```python
from build123d import *

# Parameters (mm, degrees)
EXTRUDE_1_DEPTH     = 8
SKETCH_2_R          = 1.5
CUT_EXTRUDE_1_DEPTH = 13.074353161
CHAMFER_1_SIZE      = 2


with BuildPart() as part:
    # ｽｹｯﾁ1 → ﾎﾞｽ - 押し出し1 (new body)
    with BuildSketch(Plane.XY):
        Polygon((-6.990630221, 0), (-3.009369779, 0), (-1.990630221, -2.4), (1.990630221, -2.4), (3.009369779, 0), (6.990630221, 0), (8.009369779, -2.4), (8.009369779, -4.2), (-8.009369779, -4.2), (-8.009369779, -2.4), align=None)
    extrude(amount=EXTRUDE_1_DEPTH)

    # ｽｹｯﾁ2 → ｶｯﾄ - 押し出し1 (cut, through all)
    with BuildSketch(Plane(origin=(0, 0, 0), x_dir=(1, 0, 0), z_dir=(0, 1, 0))):
        with Locations(Location((-5, -4, 0), (0, 0, 180))):
            Circle(SKETCH_2_R)
        with Locations(Location((5, -4, 0), (0, 0, 180))):
            Circle(SKETCH_2_R)
    extrude(amount=-CUT_EXTRUDE_1_DEPTH, mode=Mode.SUBTRACT)

    # 面取り1
    # the kernel refuses this chamfer: 2 mm, written as the material it takes off along each edge
    with BuildSketch(Plane(origin=(-5, -4.2, 4), x_dir=(-1, 0, 0), z_dir=(0, 0, -1))) as chamfer_1_piece_1:
        Polygon((1.5, CHAMFER_1_SIZE), (1.5 + CHAMFER_1_SIZE, 0), (1.5, 0), align=None)
    revolve(axis=Axis((-5, -4.2, 4), (0, 1, 0)), mode=Mode.SUBTRACT)
    with BuildSketch(Plane(origin=(5, -4.2, 4), x_dir=(-1, 0, 0), z_dir=(0, 0, -1))) as chamfer_1_piece_2:
        Polygon((1.5 + CHAMFER_1_SIZE, 0), (1.5, CHAMFER_1_SIZE), (1.5, 0), align=None)
    revolve(axis=Axis((5, -4.2, 4), (0, 1, 0)), mode=Mode.SUBTRACT)


solid = part.part
```
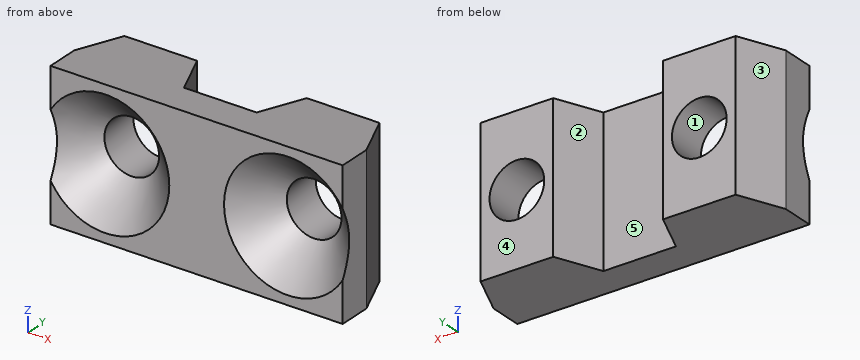
The model under review builds one solid part; all positions refer to its coordinate system, in mm. Face numbers are marked on the shaded views. A direction names the side the tool comes from. Give positions to 0.01 mm unless a question says otherwise; leave off trailing zeros. Write each loop counter-clockwise with the first axis right and the second up, starting at its lowest first coordinate (ties: lowest second). Pieces come first, ordered by that corner, then holes. Notation, with made-up numbers: M 65,19 L 91,19 A17 cw 91,31 Z; hole C 8,0.5 d5. An arc over 180 degrees is marked long. Write each question's results on one line, items separated by ' | '. Start each with the question number.
1. Insertion check: pin 1 Ø2.5 at (x, z) = (5, 4) entering from +Y; pin 2 Ø3.5 at (x, z) = (-5, 4) entering from +Y; pin 3 Ø4.5 at (x, z) = (-0.5, 5.5) entering from +Y. Each pin has a flat end and moves straight along its axis. Give the tip position at first contact, or say it passes through.
2. For the marked faces 1 and 2, list the 3-axis set-ups (+Z, -Z, +X, -X, +Y, -Y) from which the entire face can be reached by the end or side of a thin tool; tool diameter is ignored.
3. We need section C-C (y = -2). Write out the cut boundary in (x, z), and give its area (3 significant figures).
4. We need section B-B (x = 5). Write out the cut boundary in (y, z), and give its area (3 significant figures).
5. We need section D-D (y = -3.4). Write out the cut boundary in (x, z), and give its area (3 significant figures).
6. We need section A-A (y = -1.2). Write out the cut boundary in (x, z), and give its area (3 significant figures).
7. For probe 1 along Z at (x, y) = (5, -1.6); probe 2 along X at (y, z) = (-1.65, 3.5); probe 3 along X at (y, z) = (-0.15, 3.5), list the stretches that pass through material, from the lowest coordinate up. Write a range as [from, to].
8. Mouldability with a two-part tool opening along X and no side actions: class the marked faces 3, 4 and 5 as released by +X, released by -X, zero draft, split by the parting line, or undercut.
Results found:
1) pin 1: passes through | pin 2: stops at y = 0 | pin 3: stops at y = -0.61
2) face 1: +Y, -Y | face 2: +Z, -Z, +Y
3) outline: M -7.84,0 L -2.16,0 L -2.16,8 L -7.84,8 Z; M 2.16,0 L 7.84,0 L 7.84,8 L 2.16,8 Z; hole C -5,4 d3; hole C 5,4 d3 | area: 76.7 mm^2
4) outline: M -4.2,0 L 0,0 L 0,2.5 L -2.2,2.5 L -4.2,0.5 Z; M -4.2,7.5 L -2.2,5.5 L 0,5.5 L 0,8 L -4.2,8 Z | area: 17.0 mm^2
5) outline: M -8.01,0 L 8.01,0 L 8.01,8 L -8.01,8 Z; hole C -5,4 d5.4; hole C 5,4 d5.4 | area: 82.3 mm^2
6) outline: M -7.5,0 L -2.5,0 L -2.5,8 L -7.5,8 Z; M 2.5,0 L 7.5,0 L 7.5,8 L 2.5,8 Z; hole C -5,4 d3; hole C 5,4 d3 | area: 65.9 mm^2
7) probe 1: z = [0, 2.5], [5.5, 8] | probe 2: x = [-7.69, -6.41], [-3.59, -2.31], [2.31, 3.59], [6.41, 7.69] | probe 3: x = [-7.05, -6.41], [-3.59, -2.95], [2.95, 3.59], [6.41, 7.05]
8) face 3: released by -X | face 4: zero draft | face 5: undercut
